For this review, take the finished solid that the model builds, in its own axes (mm). A direction names the side the tool comes from. Round coordinates to 2 decimals unless told otherwise and drop trailing zeros. Loops run counter-clockwise (first coordinate to the right, second up) from the corner with the lowest first, then second, coordinate; pieces in that order, holes last. Notation, with made-up numbers: (29, 79) -> (51, 79) arc R11 ccw to (51, 95) -> close; hole circle Ø5 at (86.5, 1). An arc over 180 degrees is marked (long way). Write each question's results on one line, items separated by ' | '.
```python
from build123d import *

# Parameters (mm, degrees)
F0_W     = 17
F0_H     = 30
F1_DEPTH = 10
F2_W     = 10
F2_H     = 30
F3_DEPTH = 6.4
F4_R     = 2
F5_DEPTH = 25
F6_R     = 1.1
F7_DEPTH = 25
F8_W     = 10
F8_H     = 12
F9_DEPTH = 25


with BuildPart() as f1:
    # F0 (on Front) → F1 (new body)
    with BuildSketch(Plane.XZ):
        with Locations((-8.5, -15)):
            Rectangle(F0_W, F0_H)
    extrude(amount=F1_DEPTH)

    # F2 (on face) → F3 (cut)
    with BuildSketch(Plane(origin=(0, 0, 0), x_dir=(-1, 0, 0), z_dir=(0, 1, 0))):
        with Locations((5, -15)):
            Rectangle(F2_W, F2_H)
    extrude(amount=-F3_DEPTH, mode=Mode.SUBTRACT)

    # F4 (on face) → F5 (cut)
    with BuildSketch(Plane.XZ.offset(10)):
        with Locations((-13.5, -20)):
            Circle(F4_R)
    extrude(amount=-F5_DEPTH, mode=Mode.SUBTRACT)

    # F6 (on face) → F7 (cut)
    with BuildSketch(Plane.XZ.offset(10)):
        with Locations((-3, -3)):
            Circle(F6_R)
        with Locations((-3, -13)):
            Circle(F6_R)
    extrude(amount=-F7_DEPTH, mode=Mode.SUBTRACT)

    # F8 (on face) → F9 (cut)
    with BuildSketch(Plane(origin=(0, -6.4, 0), x_dir=(-1, 0, 0), z_dir=(0, 1, 0))):
        with Locations((5, -24)):
            Rectangle(F8_W, F8_H)
    extrude(amount=-F9_DEPTH, mode=Mode.SUBTRACT)


solid = f1.part
```
1. To check wall thickness, follow probe 1 along Z at (x, y) = (-13.5, -7.5); probe 2 along Z at (x, y) = (-2.5, -7.5); probe 3 along Y at (x, z) = (-3.5, -14.75). State the ranges of each line that lie inside material, in increasing order.
Values found:
probe 1: z = -30 to -22, -18 to 0 | probe 2: z = -18 to -13.98, -12.02 to -3.98, -2.02 to 0 | probe 3: y = -10 to -6.4
2. Tool access review of faces 4 (the face through (-5, -8, -18)), 5 (the face through (-14, 0, -15)): name each direction out of +Z, -Z, +X, -X, +Y, -Y from which nothing blocks a thin tool from reaching the whole face with its end or side.
Values found:
face 4: -Z, +X, +Y, -Y | face 5: +Z, -Z, +X, -X, +Y
3. Consider section D-D (y = -0.75). State the section outline as (x, z) points.
Values found:
outline: (-17, -30) -> (-10, -30) -> (-10, 0) -> (-17, 0) -> close; hole circle Ø4 at (-13.5, -20)
4. Consider section C-C (x = -3). State the section outline as (y, z) points.
Values found:
outline: (-10, -18) -> (-6.4, -18) -> (-6.4, -14.1) -> (-10, -14.1) -> close; (-10, -11.9) -> (-6.4, -11.9) -> (-6.4, -4.1) -> (-10, -4.1) -> close; (-10, -1.9) -> (-6.4, -1.9) -> (-6.4, 0) -> (-10, 0) -> close
5. Draft analysis for pull direction X (two halves, no side actions). For faces 1 (the face through (0, -8, -9)), 2 (the face through (-5, -6.4, -9)), 3 (the face through (-1.95, -8.23, -2.67)), state which applies: released by +X, released by -X, zero draft, split by the parting line, or undercut.
Values found:
face 1: released by +X | face 2: zero draft | face 3: undercut
6. For pin 1 (1 mm diameter, centred on y = -5, z = -15, fed in from +X); pin 2 (2.5 mm diameter, centred on x = -3, z = -13, fed in from +Y); pin 3 (5 mm diameter, centred on x = -13.5, z = -20, fed in from +Y); pin 4 (1.1 mm diameter, centred on x = -3, y = -8.5, fed in from -Z), all flat-tipped, find the tip position at first contact; note any pin that passes through.
Values found:
pin 1: stops at x = -10 | pin 2: stops at y = -6.4 | pin 3: stops at y = 0 | pin 4: stops at z = -18
7. Consider section A-A (z = -3). State the section outline as (x, y) points.
Values found:
outline: (-17, -10) -> (-4.1, -10) -> (-4.1, -6.4) -> (-10, -6.4) -> (-10, 0) -> (-17, 0) -> close; (-1.9, -10) -> (0, -10) -> (0, -6.4) -> (-1.9, -6.4) -> close
8. Consider section B-B (x = -13.5). State the section outline as (y, z) points, plus the area to 3 significant figures.
Values found:
outline: (-10, -30) -> (0, -30) -> (0, -22) -> (-10, -22) -> close; (-10, -18) -> (0, -18) -> (0, 0) -> (-10, 0) -> close | area: 260 mm2
